CAD build for the part. Positions are in the model's coordinates, mm. Face numbers are marked on the shaded views. A direction names the side the tool comes from. Round coordinates to 2 decimals unless told otherwise and drop trailing zeros. Order: outer loops, then holes, each group sorted by start corner. A loop starts at its lowest first (then second) coordinate and runs counter-clockwise, first axis right, second up. Notation, with made-up numbers: M 82.5,-24 L 124.5,-24 A20 ccw 124.5,-17 Z; hole C -8.75,34 d10. An arc over 180 degrees is marked long. Answer as a JSON object with one key per item and string values. Group by question number.
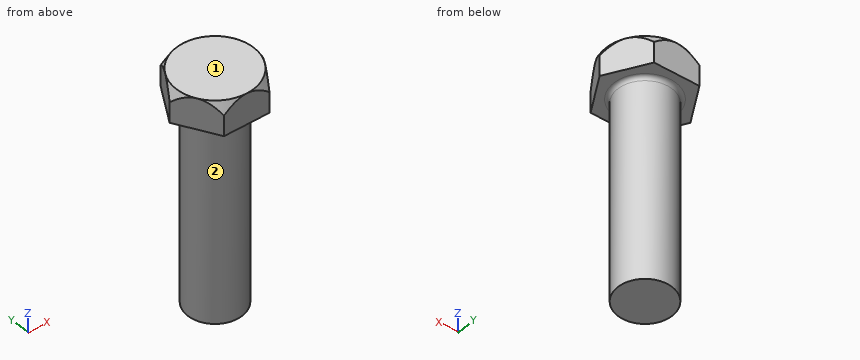
Autodesk Inventor part; units mm, degrees
ref_plane "YZ Plane" through (0, 0, 0) normal (1, 0, 0) x (0, 1, 0)
ref_plane "XZ Plane" through (0, 0, 0) normal (0, 1, 0) x (-1, 0, 0)
ref_plane "XY Plane" through (0, 0, 0) normal (0, 0, 1) x (1, 0, 0)
sketch "Sketch1" plane through (0, 0, 0) normal (0, 0, 1) x (1, 0, 0)
  line L0 (2.8868, 5) -> (5.7735, 0)
  line L1 (5.7735, 0) -> (2.8868, -5)
  line L2 (2.8868, -5) -> (-2.8868, -5)
  line L3 (-2.8868, -5) -> (-5.7735, 0)
  line L4 (-5.7735, 0) -> (-2.8868, 5)
  line L5 (-2.8868, 5) -> (2.8868, 5)
  point P0 (0, 0)
  point P1 (0, 0)
  dimension "d0" = 10
extrude "Extrusion1" add sketch "Sketch1" along normal blind 4
sketch "Sketch2" plane through (0, 0, 0) normal (0, 0, -1) x (-1, 0, 0)
  circle A0 centre (0, 0) radius 3.5
  dimension "d3" = 7
extrude "Extrusion2" add sketch "Sketch2" along normal blind 30
thread "Thread1"
fillet "Fillet1" radius 1 1 edges at (3.5, 0, -30)
fillet "Fillet2" radius 0.5 1 edges at (3.5, 0, 0)
sketch "Sketch4" plane through (0, 0, 4) normal (0, 0, 1) x (1, 0, 0)
  circle A0 centre (0, 0) radius 5
  line L0 (5.7735, 0) -> (2.8868, 5)
extrude "Extrusion4" cut sketch "Sketch4" against normal blind 30 draft 30 keep common part
properties part number "Bolt 1.0"
Item 1: Flat gauge pins, fed straight in: pin 1 Ø2 at (y, z) = (0.5, -7) entering from -X; pin 2 Ø5 at (x, y) = (3.5, -2.5) entering from -Z; pin 3 Ø6 at (y, z) = (-1, -14) entering from +X; pin 4 Ø3 at (x, z) = (2, -9.5) entering from +Y. Where does each tip first touch, or does it go through?
Item 2: Drill centre lines: line 1 (Z direction, x = 4.5, y = 0.75); line 2 (Y direction, x = -3, z = -2); line 3 (X direction, y = 0.75, z = -19.5). Where is each one in solid material? Low to high. Write a range as [from, to].
Item 3: 3-axis set-ups, long thin cutter, end or side, ignore diameter. For the marked faces 1 and 2: which of +Z, -Z, +X, -X, +Y, -Y reach the whole face in a straight line?
Item 4: Cut at A-A, the plane z = -8. Give the cut face in (x, y), and give its area (3 significant figures).
Response values:
{
 "1": {"pin 1": "x = -3.5", "pin 2": "z = -26", "pin 3": "x = 3.5", "pin 4": "y = 3.46"},
 "2": {"line 1": "[0, 4]", "line 2": "[-1.8, 1.8]", "line 3": "[-3.42, 3.42]"},
 "3": {"face 1": "+Z, +X, -X, +Y, -Y", "face 2": "-Z"},
 "4": {"outline": "C 0,0 d7", "area": "38.5 mm^2"}
}
